Verification items for the finished model (mm, model axes). A direction names the side the tool comes from. Coordinates: 2 decimals unless noted, no trailing zeros. Write each loop counter-clockwise with the first axis right and the second up, starting at its lowest first coordinate (ties: lowest second). Pieces come first, ordered by that corner, then holes. Notation, with made-up numbers: (-23.75, 14) -> (-7.75, 14) arc R33 cw to (-7.75, 53) -> close; hole circle Ø11 at (20, 3). An arc over 180 degrees is marked (long way). Answer in a Markdown table with one row per item.
```python
from build123d import *

# Parameters (mm, degrees)
SKETCH1_R           = 1.1
BOSS_EXTRUDE1_DEPTH = 1
SKETCH2_W           = 2.8
SKETCH2_H           = 5
BOSS_EXTRUDE2_DEPTH = 8
SKETCH4_W           = 2.8
SKETCH4_H           = 9
BOSS_EXTRUDE3_DEPTH = 3
SKETCH5_R           = 1.1
CUT_EXTRUDE2_DEPTH  = 100
SKETCH6_W           = 2.8
SKETCH6_H           = 8
BOSS_EXTRUDE4_DEPTH = 1
SKETCH7_W           = 3.5
SKETCH7_H           = 9
CUT_EXTRUDE3_DEPTH  = 100
CHAMFER2_SIZE       = 3
SKETCH8_W           = 10.6
SKETCH8_H           = 3
CUT_EXTRUDE4_DEPTH  = 10
BOSS_EXTRUDE5_DEPTH = 7.8
SKETCH10_W          = 10.6
SKETCH10_H          = 7
CUT_EXTRUDE5_DEPTH  = 0.5
SKETCH11_W          = 2.8
SKETCH11_H          = 4.5
BOSS_EXTRUDE6_DEPTH = 4
SKETCH12_R          = 1.1
BOSS_EXTRUDE7_DEPTH = 10.6
SKETCH13_W          = 5
SKETCH13_H          = 4.5
CUT_EXTRUDE6_DEPTH  = 10
SKETCH14_R          = 1.1
CUT_EXTRUDE7_DEPTH  = 20
FILLET1_R           = 2.5


with BuildPart() as part:
    # Sketch1 → Boss-Extrude1 (new body)
    with BuildSketch(Plane(origin=(0, 0, 0), x_dir=(1, 0, 0), z_dir=(0, 1, 0))):
        Polygon((-14.28, 13.79), (-14.28, -6.21), (-3.68, -6.21), (-3.68, 13.79), (-6.48, 13.79), (-6.48, 8.79), (-11.48, 8.79), (-11.48, 13.79), align=None)
        with Locations(Location((-8.98, 4.79, 0), (0, 0, 270))):
            Circle(SKETCH1_R, mode=Mode.SUBTRACT)
        with Locations(Location((-8.98, -1.21, 0), (0, 0, 270))):
            Circle(SKETCH1_R, mode=Mode.SUBTRACT)
    extrude(amount=BOSS_EXTRUDE1_DEPTH)

    # Sketch2 → Boss-Extrude2 (add)
    with BuildSketch(Plane(origin=(0, 1, 0), x_dir=(1, 0, 0), z_dir=(0, 1, 0))):
        with Locations((-12.88, 11.29)):
            Rectangle(SKETCH2_W, SKETCH2_H)
        with Locations((-5.08, 11.29)):
            Rectangle(SKETCH2_W, SKETCH2_H)
    extrude(amount=BOSS_EXTRUDE2_DEPTH)

    # Sketch4 → Boss-Extrude3 (add)
    with BuildSketch(Plane(origin=(0, 0, -13.79), x_dir=(-1, 0, 0), z_dir=(0, 0, -1))):
        with Locations((5.08, 4.5)):
            Rectangle(SKETCH4_W, SKETCH4_H)
        with Locations((12.88, 4.5)):
            Rectangle(SKETCH4_W, SKETCH4_H)
    extrude(amount=BOSS_EXTRUDE3_DEPTH)

    # Sketch5 → Cut-Extrude2 (cut)
    with BuildSketch(Plane(origin=(-3.68, 0, 0), x_dir=(0, 0, -1), z_dir=(1, 0, 0))):
        with Locations((14.29, 7.5)):
            Circle(SKETCH5_R)
    extrude(amount=-CUT_EXTRUDE2_DEPTH, mode=Mode.SUBTRACT)

    # Sketch6 → Boss-Extrude4 (add)
    with BuildSketch(Plane(origin=(0, 9, 0), x_dir=(1, 0, 0), z_dir=(0, 1, 0))):
        with Locations((-12.88, 12.79)):
            Rectangle(SKETCH6_W, SKETCH6_H)
        with Locations((-5.08, 12.79)):
            Rectangle(SKETCH6_W, SKETCH6_H)
    extrude(amount=BOSS_EXTRUDE4_DEPTH)

    # Sketch7 → Cut-Extrude3 (cut)
    with BuildSketch(Plane(origin=(-3.68, 0, 0), x_dir=(0, 0, -1), z_dir=(1, 0, 0))):
        with Locations((10.54, 5.5)):
            Rectangle(SKETCH7_W, SKETCH7_H)
    extrude(amount=-CUT_EXTRUDE3_DEPTH, mode=Mode.SUBTRACT)

    # Chamfer2
    chamfer2_edges = [part.edges().sort_by_distance(p)[0] for p in [
        (-5.08, 1, -12.29),
        (-12.88, 1, -12.29),
    ]]
    chamfer(chamfer2_edges, length=CHAMFER2_SIZE)

    # Sketch8 → Cut-Extrude4 (cut)
    with BuildSketch(Plane(origin=(0, 1, 0), x_dir=(1, 0, 0), z_dir=(0, 1, 0))):
        with Locations((-8.98, -4.71)):
            Rectangle(SKETCH8_W, SKETCH8_H)
    extrude(amount=-CUT_EXTRUDE4_DEPTH, mode=Mode.SUBTRACT)

    # Sketch9 → Boss-Extrude5 (add)
    with BuildSketch(Plane(origin=(-11.48, 0, 0), x_dir=(0, 0, -1), z_dir=(1, 0, 0))):
        Polygon((8.79, 1), (9.29, 1), (12.29, 4), (16.79, 4), (16.79, 0), (8.79, 0), align=None)
    extrude(amount=BOSS_EXTRUDE5_DEPTH)

    # Sketch10 → Cut-Extrude5 (cut)
    with BuildSketch(Plane(origin=(0, 1, 0), x_dir=(1, 0, 0), z_dir=(0, 1, 0))):
        with Locations((-8.98, 3.79)):
            Rectangle(SKETCH10_W, SKETCH10_H)
    extrude(amount=-CUT_EXTRUDE5_DEPTH, mode=Mode.SUBTRACT)

    # Sketch11 → Boss-Extrude6 (add)
    with BuildSketch(Plane(origin=(0, 10, 0), x_dir=(1, 0, 0), z_dir=(0, 1, 0))):
        with Locations((-12.88, 14.54)):
            Rectangle(SKETCH11_W, SKETCH11_H)
        with Locations((-5.08, 14.54)):
            Rectangle(SKETCH11_W, SKETCH11_H)
    extrude(amount=BOSS_EXTRUDE6_DEPTH)

    # Sketch12 → Boss-Extrude7 (add)
    with BuildSketch(Plane(origin=(-3.68, 0, 0), x_dir=(0, 0, -1), z_dir=(1, 0, 0))):
        with Locations((14.29, 7.5)):
            Circle(SKETCH12_R)
    extrude(amount=-BOSS_EXTRUDE7_DEPTH)

    # Sketch13 → Cut-Extrude6 (cut)
    with BuildSketch(Plane(origin=(0, 14, 0), x_dir=(1, 0, 0), z_dir=(0, 1, 0))):
        with Locations((-8.98, 14.54)):
            Rectangle(SKETCH13_W, SKETCH13_H)
    extrude(amount=-CUT_EXTRUDE6_DEPTH, mode=Mode.SUBTRACT)

    # Sketch14 → Cut-Extrude7 (cut)
    with BuildSketch(Plane(origin=(-3.68, 0, 0), x_dir=(0, 0, -1), z_dir=(1, 0, 0))):
        with Locations((14.54, 11.5)):
            Circle(SKETCH14_R)
    extrude(amount=-CUT_EXTRUDE7_DEPTH, mode=Mode.SUBTRACT)

    # Fillet1
    # the kernel refuses this fillet: 2.5 mm, written as the material it takes off along each edge
    with BuildSketch(Plane(origin=(-20.53, 14, -16.79), x_dir=(0, 0, 1), z_dir=(1, 0, 0)), Plane(origin=(-12.73, 14, -12.29), x_dir=(0, -1, 0), z_dir=(1, 0, 0)), Plane(origin=(2.57, 14, -16.79), x_dir=(0, -1, 0), z_dir=(-1, 0, 0))) as fillet1_piece_1:
        with BuildLine():
            CenterArc((FILLET1_R, FILLET1_R), FILLET1_R, 180, 90)
            Line((0, FILLET1_R), (0, 0))
            Line((0, 0), (FILLET1_R, 0))
        make_face()
    extrude(amount=15.3, mode=Mode.SUBTRACT)
    with BuildSketch(Plane(origin=(-5.23, 14, -12.29), x_dir=(0, -1, 0), z_dir=(-1, 0, 0))) as fillet1_piece_2:
        with BuildLine():
            CenterArc((FILLET1_R, -FILLET1_R), FILLET1_R, 90, 90)
            Line((0, -FILLET1_R), (0, 0))
            Line((0, 0), (FILLET1_R, 0))
        make_face()
    extrude(amount=15.3, mode=Mode.SUBTRACT)


solid = part.part
```
1. Sectioned sample at C-C, the plane x = -8.98. Record the cut outline in (y, z), and give its area (3 significant figures).
Findings below:
| item | result |
|---|---|
| outline | (0, -16.79) -> (4, -16.79) -> (4, -12.29) -> (1, -9.29) -> (1, -7.29) -> (0.5, -7.29) -> (0.5, -5.89) -> (0, -5.89) -> close; (0, -3.69) -> (0.5, -3.69) -> (0.5, -0.29) -> (1, -0.29) -> (1, 0.11) -> (0, 0.11) -> close; (0, 2.31) -> (1, 2.31) -> (1, 3.21) -> (0, 3.21) -> close |
| area | 31.2 mm² |
2. Access from +Z, -Z, +X, -X, +Y, -Y to the whole of each face (thin tool, end or side, straight path). Record for faces 1 (the face through (-11.48, 8, -15)), 2 (the face through (-9, 0.5, -3)), 3 (the face through (-9, 1, -8)).
Findings below:
| item | result |
|---|---|
| face 1 | +Z, -Z, +Y |
| face 2 | +X, -X, +Y |
| face 3 | +Z, +X, -X, +Y |
3. Release check for a two-part mould opening along X. For faces 4 (the face through (-3.68, 5, -13)), 5 (the face through (-6.48, 8, -15)), 6 (the face through (-9, 0, -7)) record: released by +X, released by -X, zero draft, split by the parting line, or undercut.
Findings below:
| item | result |
|---|---|
| face 4 | released by +X |
| face 5 | undercut |
| face 6 | zero draft |
4. Go/stop test with flat-tipped pins: pin 1 (4 mm diameter, centred on x = -6.5, z = 0.5, fed in from +Y); pin 2 (1.3 mm diameter, centred on x = -9.5, z = -13.5, fed in from +Y); pin 3 (5 mm diameter, centred on x = -9.5, y = 4, fed in from +Z). Record where each tip stops, or that it passes through.
Findings below:
| item | result |
|---|---|
| pin 1 | stops at y = 1 |
| pin 2 | stops at y = 4 |
| pin 3 | stops at z = -9.79 |
5. Sectioned sample at B-B, the plane z = -4.79. Record the cut outline in (x, y), and give its area (3 significant figures).
Findings below:
| item | result |
|---|---|
| outline | (-14.28, 0) -> (-10.08, 0) -> (-10.08, 0.5) -> (-14.28, 0.5) -> close; (-7.88, 0) -> (-3.68, 0) -> (-3.68, 0.5) -> (-7.88, 0.5) -> close |
| area | 4.20 mm² |
6. Material ranges on probe 1 along Y at (x, z) = (-4.25, -14.54); probe 2 along X at (y, z) = (0.45, 1.21); probe 3 along X at (y, z) = (13, -15), recorded low to high. Write a range as from..to.
Findings below:
| item | result |
|---|---|
| probe 1 | y = 0..10.4, 12.6..13.99 |
| probe 2 | x = -14.28..-10.08, -7.88..-3.68 |
| probe 3 | x = -14.28..-11.48, -6.48..-3.68 |
7. Sectioned sample at D-D, the plane x = -13.5. Record the cut outline in (y, z).
Findings below:
| item | result |
|---|---|
| outline | (0, -16.79) -> (11.5, -16.79) arc R2.5 ccw to (13.99, -14.54) arc R2.5 ccw to (11.5, -12.29) -> (4, -12.29) -> (1, -9.29) -> (1, -7.29) -> (0.5, -7.29) -> (0.5, -0.29) -> (1, -0.29) -> (1, 3.21) -> (0, 3.21) -> close; hole circle Ø2.2 at (11.5, -14.54) |
8. Sectioned sample at A-A, the plane y = 6.25. Record the cut outline in (x, z), and give its area (3 significant figures).
Findings below:
| item | result |
|---|---|
| outline | (-14.28, -16.79) -> (-11.48, -16.79) -> (-11.48, -12.29) -> (-14.28, -12.29) -> close; (-6.48, -16.79) -> (-3.68, -16.79) -> (-3.68, -12.29) -> (-6.48, -12.29) -> close |
| area | 25.2 mm² |
